from build123d import *

# Parameters (mm, degrees)
F2_W         = 65.4981237411
F2_H         = 65.4981237411
F2_H_2       = 68.2687636971
F3_DEPTH     = 101.6
F4_R         = 44.45
F5_DEPTH     = 63.5
F6_T         = 3.175
F6_T3_DEPTH  = 49.1841427403
F6_T5_DEPTH  = 102.8165560233
F6_T7_DEPTH  = 49.1841427403
F6_T9_DEPTH  = 49.1841427403
F6_T11_DEPTH = 49.1841427403


# Not quite as in the source:
# - a shell that OpenCascade refuses in one call is made with other operations: the cavity is built on its own and cut out


with BuildPart() as f1:
    # F0 (on Front) → F1 (revolve)
    with BuildSketch(Plane.XZ):
        with BuildLine():
            Line((0, 101.6), (0, 0))
            Line((0, 0), (7.7969783843, 17.828155983))
            add(Edge.make_bspline(
                [(7.7969783843, 17.828155983), (14.8930814395, 34.0537277243), (13.801273804, 64.5218843491), (36.8201349812, 89.6629422756), (44.45, 92.7033537653), (44.45, 101.6)],
                knots=[0, 0, 0, 0, 0.4271461897, 0.75929401, 1, 1, 1, 1], degree=3))
            Line((44.45, 101.6), (0, 101.6))
        make_face()
    revolve(axis=Axis((0, 0, 50.8), (0, 0, -1)))

    # F2 (on Top) → F3 (cut, through all)
    with BuildSketch(Plane.XY):
        with Locations((-34.3365618706, -34.3365618706)):
            Rectangle(F2_W, F2_H)
        with Locations((34.3365618706, 35.7218818486)):
            Rectangle(F2_W, F2_H_2)
        with Locations((-34.3365618706, 35.7218818486)):
            Rectangle(F2_W, F2_H_2)
        with Locations((34.3365618706, -34.3365618706)):
            Rectangle(F2_W, F2_H)
    extrude(amount=F3_DEPTH, mode=Mode.SUBTRACT)

    # F4 (on face) → F5 (join)
    with BuildSketch(Plane.XY.offset(101.6)):
        Circle(F4_R)
    extrude(amount=F5_DEPTH)

    # F6: shell of thickness 3.175, made by hand


with BuildPart() as f6_core1:
    # F6_t2: copy of F1
    add(f1.part)

    # the walls: a layer under each face that stays
    f6_faces = [f6_core1.faces().sort_by_distance(p)[0] for p in [
        (22.6899295983, 0, 71.3288999003),
        (-44.45, 0, 133.35),
        (8.7265237901, 1.5875, 85.5222406628),
        (-3.8984891922, 0, 8.9140779915),
        (23.0045713702, -1.5875, 85.5222406628),
        (23.0045713702, 23.0045713702, 101.6),
        (0, 22.6899295983, 71.3288999003),
        (-23.0045713702, 23.0045713702, 101.6),
        (-22.6899295983, 0, 71.3288999003),
        (-23.0045713702, -23.0045713702, 101.6),
        (0, -22.6899295983, 71.3288999003),
        (23.0045713702, -23.0045713702, 101.6),
        (1.5875, 23.0045713702, 85.5222406628),
        (1.5875, -8.7265237901, 85.5222406628),
        (-1.5875, -23.0045713702, 85.5222406628),
        (-8.7265237901, -1.5875, 85.5222406628),
        (-23.0045713702, 1.5875, 85.5222406628),
        (-1.5875, 8.7265237901, 85.5222406628),
    ]]
    thicken(f6_faces, amount=-F6_T, mode=Mode.SUBTRACT)

    # F6_s4 → F6_t3 (cut)
    with BuildSketch(Plane.YZ.offset(-1.5875)):
        Polygon((1.61925, 101.56825), (-1.5875, 101.6), (-1.5875, 104.775), (1.5875, 104.775), align=None)
        Polygon((-1.61925, 101.56825), (1.5875, 101.6), (1.5875, 104.775), (-1.5875, 104.775), align=None)
    extrude(amount=F6_T3_DEPTH, mode=Mode.SUBTRACT)

    # F6_s6 → F6_t5 (cut)
    with BuildSketch(Plane.XY.offset(1.9584439767)):
        Polygon((1.61925, 1.61925), (1.5875, -1.5875), (-1.5875, -1.5875), (-1.5875, 1.5875), align=None)
        Polygon((1.61925, -1.61925), (1.5875, 1.5875), (-1.5875, 1.5875), (-1.5875, -1.5875), align=None)
        Polygon((-1.61925, -1.61925), (1.5875, -1.5875), (1.5875, 1.5875), (-1.5875, 1.5875), align=None)
        Polygon((-1.61925, 1.61925), (-1.5875, -1.5875), (1.5875, -1.5875), (1.5875, 1.5875), align=None)
    extrude(amount=F6_T5_DEPTH, mode=Mode.SUBTRACT)

    # F6_s8 → F6_t7 (cut)
    with BuildSketch(Plane.XZ.offset(-47.5966427403)):
        Polygon((1.61925, 101.56825), (1.5875, 104.775), (-1.5875, 104.775), (-1.5875, 101.6), align=None)
        Polygon((-1.61925, 101.56825), (-1.5875, 104.775), (1.5875, 104.775), (1.5875, 101.6), align=None)
    extrude(amount=F6_T7_DEPTH, mode=Mode.SUBTRACT)

    # F6_s10 → F6_t9 (cut)
    with BuildSketch(Plane.YZ.offset(-47.5966427403)):
        Polygon((1.61925, 101.56825), (1.5875, 104.775), (-1.5875, 104.775), (-1.5875, 101.6), align=None)
        Polygon((-1.61925, 101.56825), (-1.5875, 104.775), (1.5875, 104.775), (1.5875, 101.6), align=None)
    extrude(amount=F6_T9_DEPTH, mode=Mode.SUBTRACT)

    # F6_s12 → F6_t11 (cut)
    with BuildSketch(Plane.XZ.offset(-1.5875)):
        Polygon((-1.61925, 101.56825), (-1.5875, 104.775), (1.5875, 104.775), (1.5875, 101.6), align=None)
        Polygon((1.61925, 101.56825), (1.5875, 104.775), (-1.5875, 104.775), (-1.5875, 101.6), align=None)
    extrude(amount=F6_T11_DEPTH, mode=Mode.SUBTRACT)


with BuildPart() as f1_1:
    add(f1.part)

    # what is left inside the walls is the cavity
    f6_cavity = [f6_core1.part.solids().sort_by_distance(p)[0] for p in [
        (-41.24325, 0, 144.991667),
    ]]
    add(f6_cavity, mode=Mode.SUBTRACT)


solid = f1_1.part
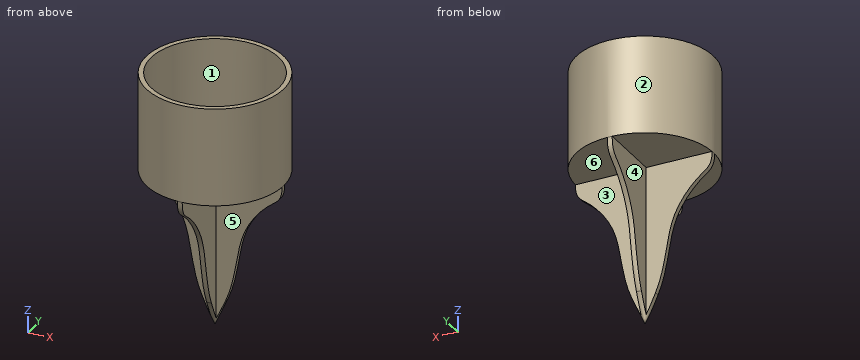
Can you work these out from the model? Positions are in its coordinate system, mm. Face numbers are marked on the shaded views. A direction names the side the tool comes from. Coordinates: 2 decimals unless noted, no trailing zeros. Write each loop counter-clockwise with the first axis right and the second up, starting at its lowest first coordinate (ties: lowest second). Pieces come first, ordered by that corner, then holes.
Q1. For P1, Ø21.5, axis at x = -29.5, z = 75.5, coming from the +Y side; P2, Ø5, axis at x = 18, y = -35.5, coming from the -Z side; P3, Ø5, axis at y = -23.5, z = 131, coming from the +X side, each with a flat end and sliding along its axis, tell me the tip position at first contact or that it passes through.
Results found:
P1: stops at y = 1.59
P2: stops at z = 101.6
P3: stops at x = 39.18
Q2. Which directions (+Z, -Z, +X, -X, +Y, -Y) give clear straight access to the entire face, cutting with the end or side of a thin tool? Please do the marked faces 4, 5 and 6.
Results found:
face 4: -Z, -X, +Y
face 5: -Z, +X, -Y
face 6: -Z, +X, +Y
Q3. Imagine slicing it at A-A, the plane z = 139. List the corners of the cut face in (x, y) for me (3 decimals).
Results found:
outline: circle Ø88.9 at (0, 0); hole circle Ø82.55 at (0, 0)
Q4. Please list where these lines run through material, in increasing order: L1, parallel to Y at x = 0, z = 134 (3 decimals); L2, parallel to Y at x = -28, z = 93; L3, parallel to Z at x = -32, y = -29.
Results found:
L1: y = -44.45 to -41.275, 41.275 to 44.45
L2: y = -1.59 to 1.59
L3: z = 101.6 to 165.1
Q5. If we mould it in two halves opening along X, with no side actions, what happens to the marked faces 1, 2 and 3? For each: +X half, -X half, draft (parallel to the pull), parting line (faces both ways), or undercut.
Results found:
face 1: undercut
face 2: parting line
face 3: draft
